Part model, mm, in its own coordinate system. Face numbers are marked on the shaded views. A direction names the side the tool comes from. Coordinates: 2 decimals unless noted, no trailing zeros. Loops run counter-clockwise (first coordinate to the right, second up) from the corner with the lowest first, then second, coordinate; pieces in that order, holes last. Notation, with made-up numbers: (56.25, 69.5) -> (94.25, 69.5) arc R23 ccw to (94.25, 102.5) -> close; hole circle Ø1 at (14, 49.25). An arc over 180 degrees is marked (long way). One line per question, with ' | ' between items. Start each with the question number.
1) Cut at C-C (y = 35). List the corners of the cut face in (x, z), plus the area to 3 significant figures.
2) Cut at A-A (x = 22.2). List the corners of the cut face in (y, z), plus the area to 3 significant figures.
3) 3-axis set-ups, long thin cutter, end or side, ignore diameter. For the marked faces 1 and 2: which of +Z, -Z, +X, -X, +Y, -Y reach the whole face in a straight line?
4) Cut at D-D (z = 5). Count the separate pieces of the cut face and the enclosed holes in it, plus the area to 3 significant figures.
5) Drop flat-ended pins along their axis: pin 1 (3 mm diameter, centred on x = -8, z = -14.5, fed in from +Y); pin 2 (10 mm diameter, centred on x = -91.5, y = 28.5, fed in from -Z). Give the stop position or say it passes through.
6) Probe L1, parallel to Y at x = -17.5, z = 2.25; L2, parallel to Y at x = 8.5, z = -10.25; L3, parallel to Z at x = -67, y = 38. List the from-to ranges inside material, lowest first. Write a range as from..to.
7) Cut at B-B (y = 62.2). List the corners of the cut face in (x, z), plus the area to 3 significant figures.
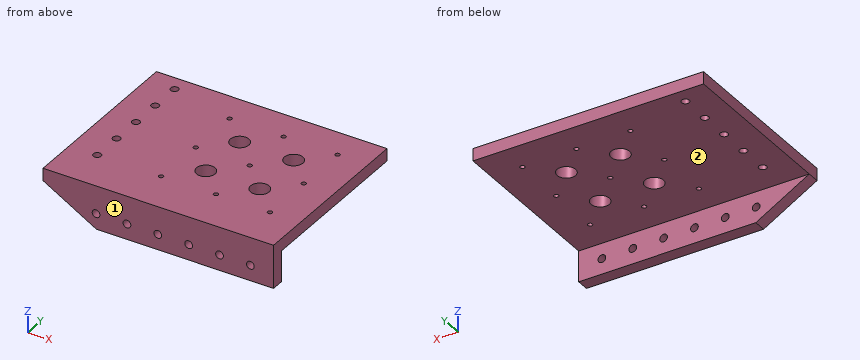
from build123d import *

# Parameters (mm, degrees)
SKETCH1_W           = 109.4
SKETCH1_H           = 109.4
SKETCH1_W_2         = 79.4
SKETCH1_H_2         = 79.4
SKETCH1_R           = 6
SKETCH1_R_2         = 1.5
BOSS_EXTRUDE1_DEPTH = 8
SKETCH2_W           = 40
SKETCH2_H           = 8
BOSS_EXTRUDE2_DEPTH = 109.4
SKETCH4_R           = 2.5
CUT_EXTRUDE1_DEPTH  = 25
SKETCH5_W           = 149.4
SKETCH5_H           = 8
SKETCH5_H_2         = 20
BOSS_EXTRUDE3_DEPTH = 8
CUT_EXTRUDE2_DEPTH  = 37
SKETCH7_R           = 2.5
CUT_EXTRUDE3_DEPTH  = 10


with BuildPart() as part:
    # Sketch1 → Boss-Extrude1 (new body)
    # profile 1 of 2: a face of its own
    with BuildSketch(Plane.XY):
        with Locations((-17.5, 17.5)):
            Rectangle(SKETCH1_W, SKETCH1_H)
        with Locations((-17.5, 17.5)):
            Rectangle(SKETCH1_W_2, SKETCH1_H_2, mode=Mode.SUBTRACT)
    # profile 2 of 2: a face of its own
    with BuildSketch(Plane.XY):
        with Locations((-17.5, 17.5)):
            Rectangle(SKETCH1_W_2, SKETCH1_H_2)
        with Locations((-35, 0)):
            Circle(SKETCH1_R, mode=Mode.SUBTRACT)
        Circle(SKETCH1_R, mode=Mode.SUBTRACT)
        with Locations((0, 35)):
            Circle(SKETCH1_R, mode=Mode.SUBTRACT)
        with Locations((-35, 35)):
            Circle(SKETCH1_R, mode=Mode.SUBTRACT)
        with Locations((-52.809903828, -17.809903828)):
            Circle(SKETCH1_R_2, mode=Mode.SUBTRACT)
        with Locations((-17.5, -17.5)):
            Circle(SKETCH1_R_2, mode=Mode.SUBTRACT)
        with Locations((17.5, -17.5)):
            Circle(SKETCH1_R_2, mode=Mode.SUBTRACT)
        with Locations((17.5, 17.5)):
            Circle(SKETCH1_R_2, mode=Mode.SUBTRACT)
        with Locations((-17.5, 17.5)):
            Circle(SKETCH1_R_2, mode=Mode.SUBTRACT)
        with Locations((-52.5, 17.5)):
            Circle(SKETCH1_R_2, mode=Mode.SUBTRACT)
        with Locations((17.5, 52.5)):
            Circle(SKETCH1_R_2, mode=Mode.SUBTRACT)
        with Locations((-17.5, 52.5)):
            Circle(SKETCH1_R_2, mode=Mode.SUBTRACT)
        with Locations((-52.5, 52.5)):
            Circle(SKETCH1_R_2, mode=Mode.SUBTRACT)
    extrude(amount=BOSS_EXTRUDE1_DEPTH)

    # Sketch2 → Boss-Extrude2 (add)
    with BuildSketch(Plane(origin=(0, 72.2, 0), x_dir=(1, 0, 0), z_dir=(0, 1, 0))):
        with Locations((-92.2, -4)):
            Rectangle(SKETCH2_W, SKETCH2_H)
    extrude(amount=-BOSS_EXTRUDE2_DEPTH)

    # Sketch4 → Cut-Extrude1 (cut)
    with BuildSketch(Plane(origin=(0, 0, 0), x_dir=(-1, 0, 0), z_dir=(0, 0, -1))):
        with Locations((94.2, 62.2)):
            Circle(SKETCH4_R)
        with Locations((94.2, 42.2)):
            Circle(SKETCH4_R)
        with Locations((94.2, 22.2)):
            Circle(SKETCH4_R)
        with Locations((94.2, 2.2)):
            Circle(SKETCH4_R)
        with Locations((94.2, -17.8)):
            Circle(SKETCH4_R)
    extrude(amount=-CUT_EXTRUDE1_DEPTH, mode=Mode.SUBTRACT)

    # Sketch5 → Boss-Extrude3 (add)
    with BuildSketch(Plane.XZ.offset(37.2)):
        with Locations((-37.5, 4)):
            Rectangle(SKETCH5_W, SKETCH5_H)
        with Locations((-37.5, -10)):
            Rectangle(SKETCH5_W, SKETCH5_H_2)
    extrude(amount=BOSS_EXTRUDE3_DEPTH)

    # Sketch6 → Cut-Extrude2 (cut)
    with BuildSketch(Plane(origin=(0, -37.2, 0), x_dir=(1, 0, 0), z_dir=(0, 1, 0))):
        Polygon((-112.2, 0), (-77.558983849, 20), (-112.2, 20), align=None)
    extrude(amount=-CUT_EXTRUDE2_DEPTH, mode=Mode.SUBTRACT)

    # Sketch7 → Cut-Extrude3 (cut)
    with BuildSketch(Plane(origin=(0, -37.2, 0), x_dir=(1, 0, 0), z_dir=(0, 1, 0))):
        with Locations(Location((22.2, 10, 0), (0, 0, 180))):
            Circle(SKETCH7_R)
        with Locations(Location((2.2, 10, 0), (0, 0, 180))):
            Circle(SKETCH7_R)
        with Locations(Location((-17.8, 10, 0), (0, 0, 180))):
            Circle(SKETCH7_R)
        with Locations(Location((-37.8, 10, 0), (0, 0, 180))):
            Circle(SKETCH7_R)
        with Locations(Location((-57.8, 10, 0), (0, 0, 180))):
            Circle(SKETCH7_R)
        with Locations(Location((-77.8, 10, 0), (0, 0, 180))):
            Circle(SKETCH7_R)
    extrude(amount=-CUT_EXTRUDE3_DEPTH, mode=Mode.SUBTRACT)


solid = part.part
Reported:
1) outline: (-112.2, 0) -> (-41, 0) -> (-41, 8) -> (-112.2, 8) -> close; (-29, 0) -> (-6, 0) -> (-6, 8) -> (-29, 8) -> close; (6, 0) -> (37.2, 0) -> (37.2, 8) -> (6, 8) -> close | area: 1,000 mm²
2) outline: (-45.2, -20) -> (-37.2, -20) -> (-37.2, -12.5) -> (-45.2, -12.5) -> close; (-45.2, -7.5) -> (-37.2, -7.5) -> (-37.2, 0) -> (72.2, 0) -> (72.2, 8) -> (-45.2, 8) -> close | area: 1,060 mm²
3) face 1: +Z, -Z, +X, -X, -Y | face 2: -Z, +X, -X, +Y
4) separate pieces: 1 | enclosed holes: 18 | area: 16,900 mm²
5) pin 1: stops at y = -37.2 | pin 2: stops at z = 0
6) L1: y = -45.2..-19, -16..16, 19..51, 54..72.2 | L2: y = -45.2..-37.2 | L3: z = 0..8
7) outline: (-112.2, 0) -> (-96.7, 0) -> (-96.7, 8) -> (-112.2, 8) -> close; (-91.7, 0) -> (37.2, 0) -> (37.2, 8) -> (-91.7, 8) -> close | area: 1,160 mm²
